Geometry: see drawing. Coordinates: mm, zero at the bounding-box minimum. A direction names the side the tool comes from. Give positions to 0.01 mm unless a question says otherwise; leave off trailing zeros. Write each loop counter-clockwise with the first axis right and the second up, starting at its lowest first coordinate (ties: lowest second). Pieces come first, ordered by that corner, then holes. Notation, with made-up numbers: (32, -39) -> (84, -39) arc R13 cw to (84, -29) -> close; hole circle Ø4 at (72, 38.5). An arc over 180 degrees is marked (long way). Answer as a JSON object with one key per item and string values. Group by question number.
Item 1: Section query C-C on y = 13. Return the cut outline in (x, z), plus the area to 3 significant figures.
Item 2: Ray query, probe 1 along Z at (x, y) = (53, 5); probe 2 along X at (y, z) = (19, 1.5); probe 3 along X at (y, z) = (12, 15.5). Return the intervals inside material, ascending. Write a range as from..to.
Item 3: Section query A-A on x = 56. Return the cut outline in (y, z).
Item 4: First-contact query: pin 1 Ø6 at (x, y) = (15, 15) entering from +Z; pin 2 Ø8.5 at (y, z) = (11, 7.5) entering from -X; pin 3 Ø16 at (x, y) = (65, 15) entering from +Z; pin 4 Ø3 at (y, z) = (5, 8.5) entering from +X. Flat tips, straight axial feed; report the tip coordinate or a pass-through.
Item 5: Section query B-B on z = 18.5. Return the cut outline in (x, y), plus the area to 3 significant figures.
Item 6: Section query D-D on x = 19. Return the cut outline in (y, z).
Item 7: Access query for the marked faces 5, 6 and 7. Directions: +Z, -Z, +X, -X, +Y, -Y. A direction counts if a zero-diameter tool reaches every point of the face in a straight line with its end or side. Return the directions, or none.
Item 8: Pull-direction query (X, two-part tool) for the marked faces 1, 2, 3 and 4; classes: pulls with the +X half, pulls with the -X half, needs draft (parallel to the pull), parting line crosses it, or undercut.
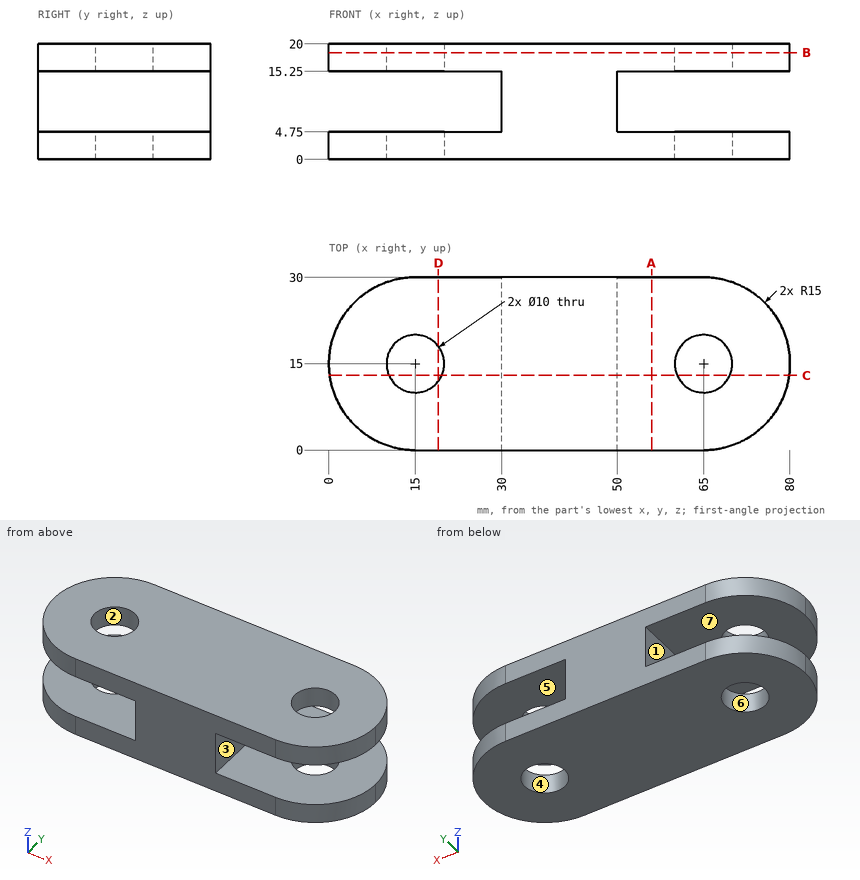
Worked answers:
{
 "1": {"outline": "(0.13, 0) -> (10.42, 0) -> (10.42, 4.75) -> (0.13, 4.75) -> close; (0.13, 15.25) -> (10.42, 15.25) -> (10.42, 20) -> (0.13, 20) -> close; (19.58, 0) -> (60.42, 0) -> (60.42, 4.75) -> (50, 4.75) -> (50, 15.25) -> (60.42, 15.25) -> (60.42, 20) -> (19.58, 20) -> (19.58, 15.25) -> (30, 15.25) -> (30, 4.75) -> (19.58, 4.75) -> close; (69.58, 0) -> (79.87, 0) -> (79.87, 4.75) -> (69.58, 4.75) -> close; (69.58, 15.25) -> (79.87, 15.25) -> (79.87, 20) -> (69.58, 20) -> close", "area": "793 mm^2"},
 "2": {"probe 1": "0..4.75, 15.25..20", "probe 2": "0.54..12, 18..62, 68..79.46", "probe 3": "0.3..11, 19..61, 69..79.7"},
 "3": {"outline": "(0, 0) -> (30, 0) -> (30, 4.75) -> (0, 4.75) -> close; (0, 15.25) -> (30, 15.25) -> (30, 20) -> (0, 20) -> close"},
 "4": {"pin 1": "through", "pin 2": "x = 0.02", "pin 3": "z = 20", "pin 4": "x = 50"},
 "5": {"outline": "(0, 15) arc R15 ccw to (15, 0) -> (65, 0) arc R15 ccw to (80, 15) arc R15 ccw to (65, 30) -> (15, 30) arc R15 ccw to start; hole circle Ø10 at (15, 15); hole circle Ø10 at (65, 15)", "area": "2,050 mm^2"},
 "6": {"outline": "(0, 0) -> (12, 0) -> (12, 4.75) -> (0, 4.75) -> close; (0, 15.25) -> (12, 15.25) -> (12, 20) -> (0, 20) -> close; (18, 0) -> (30, 0) -> (30, 4.75) -> (18, 4.75) -> close; (18, 15.25) -> (30, 15.25) -> (30, 20) -> (18, 20) -> close"},
 "7": {"face 5": "+X, +Y, -Y", "face 6": "+Z, -Z", "face 7": "-X, +Y, -Y"},
 "8": {"face 1": "pulls with the -X half", "face 2": "undercut", "face 3": "pulls with the +X half", "face 4": "undercut"}
}
